The listing builds one solid part. Answer for the finished solid, in the listing's coordinates (mm). Give positions to 0.01 mm unless a question says otherwise; leave off trailing zeros. Order: outer loops, then holes, each group sorted by start corner. A loop starts at its lowest first (then second) coordinate and runs counter-clockwise, first axis right, second up.
```python
from build123d import *

# Parameters (mm, degrees)
MASTER_SKETCH_R       = 52.451
MASTER_SKETCH_R_2     = 9.525
MASTER_SKETCH_R_3     = 45.974
MASTER_SKETCH_R_4     = 27.4955
MASTER_SKETCH_R_5     = 6.5
BOSS_EXTRUDE2_DEPTH   = 4.7625
F_5_0MM_DOWEL_HOLE1_D = 5
CIRPATTERN4_COUNT     = 4
M6_CLEARANCE_HOLE4_D  = 6.6
M8_CLEARANCE_HOLE1_D  = 9
CIRPATTERN3_COUNT     = 9
CUT_EXTRUDE2_DEPTH    = 284.948803699
CUT_EXTRUDE3_DEPTH    = 284.948803699
FILLET1_R             = 2.54


with BuildPart() as part:
    # Master Sketch → Boss-Extrude2 (new, symmetric)
    # profile 1 of 5: a face of its own
    with BuildSketch(Plane(origin=(0, 0, 0), x_dir=(1, 0, 0), z_dir=(0, 1, 0))):
        with BuildLine():
            ThreePointArc((-8.636, 127), (-36.396097826, 84.787887478), (-86.152093601, 93.552952189))
            Line((-86.152093601, 93.552952189), (-6.534964144, 18.470363023))
            ThreePointArc((-6.534964144, 18.470363023), (-3.773598517, 34.145603423), (9.525, 25.4))
            ThreePointArc((9.525, 25.4), (8.799952547, 21.754940307), (6.735192091, 18.664807909))
            Line((6.735192091, 18.664807909), (34.255961574, 46.185577392))
            ThreePointArc((34.255961574, 46.185577392), (59.945142207, 60.02346539), (89.010077776, 57.44457682))
            Line((89.010077776, 57.44457682), (207.987004211, 9.951947906))
            ThreePointArc((207.987004211, 9.951947906), (204.851852042, 25.601533276), (220.43444462, 22.148779315))
            Line((220.43444462, 22.148779315), (189.133864847, 105.44289655))
            ThreePointArc((189.133864847, 105.44289655), (188.207777178, 115.4635324), (192.51641215, 124.557840832))
            Line((192.51641215, 124.557840832), (212.800120602, 148.168522003))
            ThreePointArc((212.800120602, 148.168522003), (196.940842995, 150.353698677), (205.472725722, 163.899866417))
            Line((205.472725722, 163.899866417), (169.599038165, 163.514054819))
            ThreePointArc((169.599038165, 163.514054819), (163.800537316, 164.352688386), (158.531122559, 166.913779261))
            ThreePointArc((158.531122559, 166.913779261), (141.706259737, 175.147152322), (123.19, 177.9778))
            Line((123.19, 177.9778), (-54.61, 172.974))
            ThreePointArc((-54.61, 172.974), (-22.101472842, 159.508527158), (-8.636, 127))
        make_face()
        with Locations(Location((123.19, 116.0018, 0), (0, 0, 90))):
            Circle(MASTER_SKETCH_R, mode=Mode.SUBTRACT)
    # profile 2 of 5: a face of its own
    with BuildSketch(Plane(origin=(0, 0, 0), x_dir=(1, 0, 0), z_dir=(0, 1, 0))):
        with Locations((0, 25.4)):
            Circle(MASTER_SKETCH_R_2)
    # profile 3 of 5: a face of its own
    with BuildSketch(Plane(origin=(0, 0, 0), x_dir=(1, 0, 0), z_dir=(0, 1, 0))):
        with Locations((211.518208908, 18.79820239)):
            Circle(MASTER_SKETCH_R_2)
    # profile 4 of 5: a face of its own
    with BuildSketch(Plane(origin=(0, 0, 0), x_dir=(1, 0, 0), z_dir=(0, 1, 0))):
        with Locations((205.575158542, 154.375417219)):
            Circle(MASTER_SKETCH_R_2)
    # profile 5 of 5: a face of its own
    with BuildSketch(Plane(origin=(0, 0, 0), x_dir=(1, 0, 0), z_dir=(0, 1, 0))):
        with Locations((-54.61, 127)):
            Circle(MASTER_SKETCH_R_3)
        with Locations(Location((-54.61, 127, 0), (0, 0, 90))):
            Circle(MASTER_SKETCH_R_4, mode=Mode.SUBTRACT)
        with Locations(Location((-67.94878559, 163.648012211, 0), (0, 0, 90))):
            Circle(MASTER_SKETCH_R_5, mode=Mode.SUBTRACT)
        with Locations(Location((-41.27121441, 163.648012211, 0), (0, 0, 90))):
            Circle(MASTER_SKETCH_R_5, mode=Mode.SUBTRACT)
    extrude(amount=BOSS_EXTRUDE2_DEPTH, both=True)

    # Ø5.0mm Dowel Hole1 (through all)
    with Locations(Plane(origin=(0, 4.7625, 0), x_dir=(1, 0, 0), z_dir=(0, 1, 0))):
        with Locations((123.19, 173.1518)):
            f_5_0mm_dowel_hole1 = Hole(F_5_0MM_DOWEL_HOLE1_D / 2)

    # CirPattern4: Ø5.0mm Dowel Hole1 ×4 about axis
    cirpattern4_axis = Axis((123.19, 0, -116.0018), (0, 1, 0))
    for i in range(1, CIRPATTERN4_COUNT):
        add(f_5_0mm_dowel_hole1.rotate(cirpattern4_axis, i * 360 / CIRPATTERN4_COUNT), mode=Mode.SUBTRACT)

    # M6 Clearance Hole4 (through all)
    with Locations(Plane(origin=(0, 4.7625, 0), x_dir=(1, 0, 0), z_dir=(0, 1, 0))):
        with Locations((205.575158542, 154.375417219), (211.518208908, 18.79820239), (0, 25.4)):
            Hole(M6_CLEARANCE_HOLE4_D / 2)

    # M8 Clearance Hole1 (through all)
    with Locations(Plane(origin=(0, 4.7625, 0), x_dir=(1, 0, 0), z_dir=(0, 1, 0))):
        with Locations((-54.61, 166)):
            m8_clearance_hole1 = Hole(M8_CLEARANCE_HOLE1_D / 2)

    # CirPattern3: M8 Clearance Hole1 ×9 about axis
    cirpattern3_axis = Axis((-54.61, 0, -127), (0, 1, 0))
    for i in range(1, CIRPATTERN3_COUNT):
        add(m8_clearance_hole1.rotate(cirpattern3_axis, i * 360 / CIRPATTERN3_COUNT), mode=Mode.SUBTRACT)

    # Topology 3 → Cut-Extrude2 (cut, through all)
    with BuildSketch(Plane(origin=(0, 4.7625, 0), x_dir=(1, 0, 0), z_dir=(0, 1, 0))):
        with BuildLine():
            ThreePointArc((148.153589294, 55.823132596), (164.735029841, 65.81551406), (177.648151764, 80.239214699))
            ThreePointArc((177.648151764, 80.239214699), (183.658143307, 83.064639882), (188.900120968, 78.987300553))
            Line((188.900120968, 78.987300553), (205.194131764, 35.627233252))
            ThreePointArc((205.194131764, 35.627233252), (203.319232726, 27.16564341), (194.821264757, 25.463207079))
            Line((194.821264757, 25.463207079), (148.232551201, 44.060262413))
            ThreePointArc((148.232551201, 44.060262413), (144.236830733, 49.915140022), (148.153589294, 55.823132596))
        make_face()
        with BuildLine():
            Line((190.127076346, 136.393510988), (194.150985671, 141.077429629))
            ThreePointArc((194.150985671, 141.077429629), (195.32544691, 149.601274428), (188.044823271, 154.186883307))
            Line((188.044823271, 154.186883307), (181.870154841, 154.120476454))
            ThreePointArc((181.870154841, 154.120476454), (179.135815493, 152.500048502), (179.17593949, 149.321874737))
            ThreePointArc((179.17593949, 149.321874737), (182.248718341, 143.510354832), (184.720207534, 137.418764347))
            ThreePointArc((184.720207534, 137.418764347), (187.127250613, 135.343061567), (190.127076346, 136.393510988))
        make_face()
        with BuildLine():
            ThreePointArc((64.098067009, 143.438932802), (66.306808777, 147.765857633), (68.831828447, 151.916170194))
            ThreePointArc((68.831828447, 151.916170194), (69.209050275, 161.796201373), (60.61677272, 166.688039353))
            Line((60.61677272, 166.688039353), (-1.663792567, 164.935286301))
            ThreePointArc((-1.663792567, 164.935286301), (-9.632748017, 160.197249287), (-9.798074059, 150.927626155))
            ThreePointArc((-9.798074059, 150.927626155), (-6.09260405, 142.056636088), (-4.12477238, 132.646396384))
            ThreePointArc((-4.12477238, 132.646396384), (-0.093621954, 125.882803807), (7.651359628, 124.464488392))
            Line((7.651359628, 124.464488392), (55.659374127, 136.466492017))
            ThreePointArc((55.659374127, 136.466492017), (60.668494681, 138.996854714), (64.098067009, 143.438932802))
        make_face()
        with BuildLine():
            ThreePointArc((17.44176984, 42.84176984), (-0.146601343, 35.405008389), (-17.945313453, 42.323250142))
            Line((-17.945313453, 42.323250142), (-33.032755262, 56.551396808))
            ThreePointArc((-33.032755262, 56.551396808), (-37.018106584, 65.604842248), (-33.299725858, 74.771168898))
            Line((-33.299725858, 74.771168898), (-25.157987823, 82.912906934))
            ThreePointArc((-25.157987823, 82.912906934), (-16.98904431, 89.126755018), (-7.457826773, 92.934567826))
            Line((-7.457826773, 92.934567826), (48.48636159, 106.920614917))
            ThreePointArc((48.48636159, 106.920614917), (55.6852269, 105.854731176), (60.030376503, 100.016970919))
            ThreePointArc((60.030376503, 100.016970919), (62.745475764, 91.688999032), (66.553177874, 83.800508404))
            ThreePointArc((66.553177874, 83.800508404), (66.885503662, 75.024623751), (59.896219631, 69.707058463))
            ThreePointArc((59.896219631, 69.707058463), (42.409632623, 63.819008448), (27.520769483, 52.920769483))
            Line((27.520769483, 52.920769483), (17.44176984, 42.84176984))
        make_face()
    extrude(amount=-CUT_EXTRUDE2_DEPTH, mode=Mode.SUBTRACT)

    # Sketch29 → Cut-Extrude3 (cut, through all)
    with BuildSketch(Plane.XZ.offset(4.7625)):
        with BuildLine():
            Line((-72.305646266, -158.824345033), (-79.713448931, -165.515263569))
            ThreePointArc((-79.713448931, -165.515263569), (-70.954498766, -169.970525201), (-61.44878559, -172.462508594))
            Line((-61.44878559, -172.462508594), (-61.44878559, -163.648012211))
            ThreePointArc((-61.44878559, -163.648012211), (-70.587952655, -169.588112984), (-72.305646266, -158.824345033))
        make_face()
        with BuildLine():
            Line((-47.77121441, -163.648012211), (-47.77121441, -173.166462966))
            Line((-47.77121441, -173.166462966), (-34.77121441, -173.532320109))
            Line((-34.77121441, -173.532320109), (-34.77121441, -163.648012211))
            ThreePointArc((-34.77121441, -163.648012211), (-41.27121441, -170.148012211), (-47.77121441, -163.648012211))
        make_face()
    extrude(amount=-CUT_EXTRUDE3_DEPTH, mode=Mode.SUBTRACT)

    # Fillet1
    fillet1_edges = [part.edges().sort_by_distance(p)[0] for p in [
        (-79.713448931, 0, -165.515263569),
        (-61.44878559, 0, -172.462508594),
        (-47.77121441, 0, -173.166462966),
        (-34.77121441, 0, -173.532320109),
    ]]
    fillet(fillet1_edges, radius=FILLET1_R)


solid = part.part
```
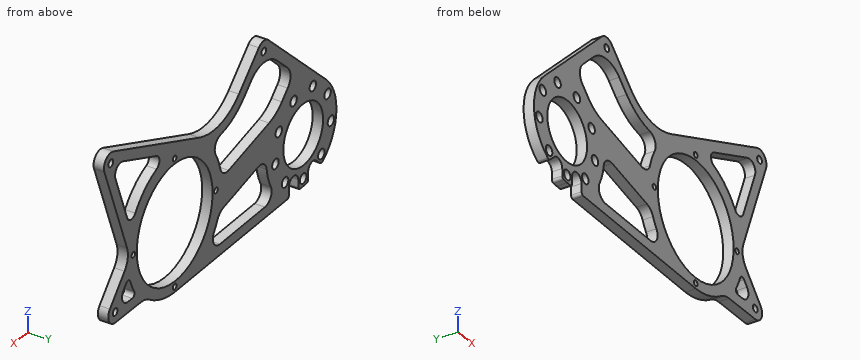
1) Find section B-B (x = 45). Write down the section's boundary in (y, z), then the cut area to 3 significant figures.
Geometry says:
outline: (-4.76, -175.78) - (4.76, -175.78) - (4.76, -166.25) - (-4.76, -166.25) - close; (-4.76, -133.8) - (4.76, -133.8) - (4.76, -106.05) - (-4.76, -106.05) - close; (-4.76, -65.08) - (4.76, -65.08) - (4.76, -54.39) - (-4.76, -54.39) - close
area: 457 mm2
2) Straight lines are drawn through the part: probe 1 along Z at (x, y) = (-9, -2.75) (3 decimals); probe 2 along X at (y, z) = (-3.75, -140.5); probe 3 along Z at (x, y) = (-22, 1.75). For each, find the intervals that lie inside material, in ascending order.
Geometry says:
probe 1: z = -174.258 to -161.15, -149.369 to -92.514, -36.86 to -20.795
probe 2: x = -98.56 to -78.56, -30.66 to -5.64, 62.2 to 76.81, 169.57 to 183.56, 193.65 to 206.21
probe 3: z = -173.89 to -111.85, -103.15 to -85.74, -46.15 to -33.05
3) Given P1, Ø3, axis at x = 180.34, z = -116, coming from the +Y side; P2, Ø4, axis at x = 44, y = 2.5, coming from the -Z side; P3, Ø1.5, axis at x = 54, y = 3.5, coming from the -Z side; P4, Ø3, axis at x = 173.5, y = 3.5, coming from the +Z side, each flat-ended and moving along its own axis, determine where each tip first touches the part or whether it passes through.
Geometry says:
P1: passes through
P2: stops at z = -175.81
P3: stops at z = -176.05
P4: stops at z = -23.12
4) Find section C-C (y = 3.25). Count the separate pieces of the cut face and the enclosed holes in it, then the cut area to 3 significant figures.
Geometry says:
separate pieces: 1
enclosed holes: 22
area: 16,700 mm2
5) Find section A-A (x = 164.5). Write down the section's boundary in (y, z), then the cut area to 3 significant figures.
Geometry says:
outline: (-4.76, -164.15) - (4.76, -164.15) - (4.76, -148.32) - (-4.76, -148.32) - close; (-4.76, -83.68) - (4.76, -83.68) - (4.76, -65.62) - (-4.76, -65.62) - close; (-4.76, -37.57) - (4.76, -37.57) - (4.76, -27.31) - (-4.76, -27.31) - close
area: 420 mm2
